```python
from build123d import *

# Parameters (mm, degrees)
SKETCH1_W           = 21.384482042
SKETCH1_H           = 82.225
SKETCH1_R           = 2
BOSS_EXTRUDE1_DEPTH = 6.35
CHAMFER1_SIZE       = 1


with BuildPart() as part:
    # Sketch1 → Boss-Extrude1 (new body)
    with BuildSketch(Plane(origin=(0, 0, 0), x_dir=(1, 0, 0), z_dir=(0, 1, 0))):
        with Locations((0, 6.1625)):
            Rectangle(SKETCH1_W, SKETCH1_H)
        with Locations(Location((0, 42.5, 0), (0, 0, 270))):
            Circle(SKETCH1_R, mode=Mode.SUBTRACT)
        with Locations(Location((0, -4.775, 0), (0, 0, 90))):
            Circle(SKETCH1_R, mode=Mode.SUBTRACT)
        with Locations(Location((0, -26.95, 0), (0, 0, 270))):
            Circle(SKETCH1_R, mode=Mode.SUBTRACT)
    extrude(amount=BOSS_EXTRUDE1_DEPTH)

    # Chamfer1
    chamfer1_edges = [part.edges().sort_by_distance(p)[0] for p in [
        (0, 6.35, -44.5),
        (0, 6.35, 34.95),
        (0, 6.35, 6.775),
        (10.692241021, 6.35, -6.1625),
        (0, 6.35, 24.95),
        (0, 6.35, -47.275),
        (-10.692241021, 6.35, -6.1625),
    ]]
    chamfer(chamfer1_edges, length=CHAMFER1_SIZE)


solid = part.part
```
Model file for the job. Use its own axes, mm. Coordinates: 2 decimals unless noted, no trailing zeros. Loops run counter-clockwise (first coordinate to the right, second up) from the corner with the lowest first, then second, coordinate; pieces in that order, holes last. Notation, with made-up numbers: (42, -30) - (96, -30) arc R22 ccw to (96, -11) - close; hole circle Ø6 at (-12, 39). An arc over 180 degrees is marked (long way). Answer as a JSON object with one key per item and string values. Group by question number.
(1) Probe line 1 along X through (y, z) = (2.55, -42.5); line 2 along Z through (x, y) = (8.75, 5.75) (3 decimals); line 3 along Y through (x, z) = (-1.75, -44). List the from-to ranges inside material, lowest first.
(2) Two-plate mould, pull along X, no slides. Class faces 1 (the face through (-10.692, 3, -6)), 2 (the face through (0, 3, -47.275)), 3 (the face through (-0.766, 2.638, 28.797)): released by +X, released by -X, zero draft, split by the parting line, or undercut.
(3) Flat gauge pin, fed straight in: pin 1 (6.5 mm diameter, centred on x = 0, z = 26.95, fed in from +Y). Where does the tip first touch, or does it go through?
(4) Cut at A-A (x = 0). Give the cut face in (y, z) (3 decimals), then the cut area to 3 significant figures.
(5) Cut at B-B (z = -42.5). Give the cut face in (x, y), then the cut area to 3 significant figures.
Geometry says:
{
 "1": {"line 1": "x = -10.69 to -2, 2 to 10.69", "line 2": "z = -46.875 to 34.55", "line 3": "y = 0 to 5.65"},
 "2": {"face 1": "released by -X", "face 2": "zero draft", "face 3": "undercut"},
 "3": {"pin 1": "stops at y = 6.35"},
 "4": {"outline": "(0, -47.275) - (5.35, -47.275) - (6.35, -46.275) - (6.35, -45.5) - (5.35, -44.5) - (0, -44.5) - close; (0, -40.5) - (5.35, -40.5) - (6.35, -39.5) - (6.35, 1.775) - (5.35, 2.775) - (0, 2.775) - close; (0, 6.775) - (5.35, 6.775) - (6.35, 7.775) - (6.35, 23.95) - (5.35, 24.95) - (0, 24.95) - close; (0, 28.95) - (5.35, 28.95) - (6.35, 29.95) - (6.35, 33.95) - (5.35, 34.95) - (0, 34.95) - close", "area": "442 mm^2"},
 "5": {"outline": "(-10.69, 0) - (-2, 0) - (-2, 5.35) - (-3, 6.35) - (-9.69, 6.35) - (-10.69, 5.35) - close; (2, 0) - (10.69, 0) - (10.69, 5.35) - (9.69, 6.35) - (3, 6.35) - (2, 5.35) - close", "area": "108 mm^2"}
}
